Read the model definition and answer for the solid it produces. Units are mm, in the model's axes. Round coordinates to 2 decimals unless told otherwise and drop trailing zeros. Loops run counter-clockwise (first coordinate to the right, second up) from the corner with the lowest first, then second, coordinate; pieces in that order, holes last. Notation, with made-up numbers: M -18.75,54.25 L 32.25,54.25 A11 cw 32.25,69.25 Z; hole C 56,34.25 d9. An arc over 180 degrees is marked long. Answer as CSV lines item,"result".
```python
from build123d import *

# Parameters (mm, degrees)
SKETCH_1_W          = 40
SKETCH_1_H          = 170
SKETCH_1_R          = 1.5
EXTRUDE_1_DEPTH     = 5
FILLET_1_R          = 5
SKETCH_2_R          = 3
CUT_EXTRUDE_1_DEPTH = 3


with BuildPart() as part:
    # 草图1 → 凸台-拉伸1 (new body)
    with BuildSketch(Plane(origin=(0, 0, 0), x_dir=(1, 0, 0), z_dir=(0, 1, 0))):
        Rectangle(SKETCH_1_W, SKETCH_1_H)
        with Locations(Location((-15, 70, 0), (0, 0, 270))):
            Circle(SKETCH_1_R, mode=Mode.SUBTRACT)
        with Locations(Location((15, 70, 0), (0, 0, 270))):
            Circle(SKETCH_1_R, mode=Mode.SUBTRACT)
        with Locations(Location((15, -10, 0), (0, 0, 270))):
            Circle(SKETCH_1_R, mode=Mode.SUBTRACT)
        with Locations(Location((-15, -10, 0), (0, 0, 270))):
            Circle(SKETCH_1_R, mode=Mode.SUBTRACT)
        with Locations(Location((12, -46, 0), (0, 0, 270))):
            Circle(SKETCH_1_R, mode=Mode.SUBTRACT)
        with Locations(Location((-12, -46, 0), (0, 0, 270))):
            Circle(SKETCH_1_R, mode=Mode.SUBTRACT)
        with Locations(Location((-12, -75, 0), (0, 0, 270))):
            Circle(SKETCH_1_R, mode=Mode.SUBTRACT)
        with Locations(Location((12, -75, 0), (0, 0, 270))):
            Circle(SKETCH_1_R, mode=Mode.SUBTRACT)
    extrude(amount=EXTRUDE_1_DEPTH)

    # 圆角1
    fillet_1_edges = [part.edges().sort_by_distance(p)[0] for p in [
        (20, 2.5, 85),
        (-20, 2.5, 85),
        (-20, 2.5, -85),
        (20, 2.5, -85),
    ]]
    fillet(fillet_1_edges, radius=FILLET_1_R)

    # 草图2 → 切除-拉伸1 (cut)
    with BuildSketch(Plane.XZ):
        with Locations(Location((-12, 75, 0), (0, 0, 270))):
            Circle(SKETCH_2_R)
        with Locations(Location((12, 75, 0), (0, 0, 270))):
            Circle(SKETCH_2_R)
        with Locations(Location((12, 46, 0), (0, 0, 270))):
            Circle(SKETCH_2_R)
        with Locations(Location((-12, 46, 0), (0, 0, 270))):
            Circle(SKETCH_2_R)
    extrude(amount=-CUT_EXTRUDE_1_DEPTH, mode=Mode.SUBTRACT)


solid = part.part
```
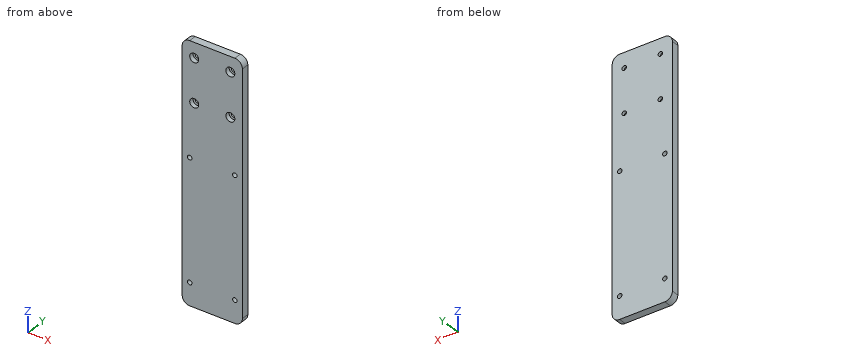
1) This flat-tipped pin is pushed along its axis until it touches: P1, Ø3, axis at x = 12.5, z = 75.5, coming from the -Y side. Where does it stop, or does it pass through?
Evaluation:
P1,"stops at y = 3"
2) Straight lines are drawn through the part: line 1 (Z direction, x = 12, y = 4); line 2 (X direction, y = 2, z = 75); line 3 (Z direction, x = 13, y = 1.85). For each, find the intervals that lie inside material, in ascending order.
Evaluation:
line 1,"z = -85 to 44.5, 47.5 to 73.5, 76.5 to 85"
line 2,"x = -20 to -15, -9 to 9, 15 to 20"
line 3,"z = -85 to 43.17, 48.83 to 72.17, 77.83 to 85"
3) Find section C-C, the plane x = 12. Give the vertices of the cut face in (y, z), then the cut area to 3 significant figures.
Evaluation:
outline,"M 0,-85 L 5,-85 L 5,44.5 L 3,44.5 L 3,43 L 0,43 Z; M 0,49 L 3,49 L 3,47.5 L 5,47.5 L 5,73.5 L 3,73.5 L 3,72 L 0,72 Z; M 0,78 L 3,78 L 3,76.5 L 5,76.5 L 5,85 L 0,85 Z"
area,"802 mm^2"
4) Find section D-D, the plane z = 75. Give the vertices of the cut face in (x, y), then the cut area to 3 significant figures.
Evaluation:
outline,"M -20,0 L -15,0 L -15,3 L -13.5,3 L -13.5,5 L -20,5 Z; M -10.5,3 L -9,3 L -9,0 L 9,0 L 9,3 L 10.5,3 L 10.5,5 L -10.5,5 Z; M 13.5,3 L 15,3 L 15,0 L 20,0 L 20,5 L 13.5,5 Z"
area,"152 mm^2"
5) Find section B-B, the plane y = 1.25. Count the separate pieces of the cut face and the enclosed holes in it, then the cut area to 3 significant figures.
Evaluation:
separate pieces,"1"
enclosed holes,"8"
area,"6,640 mm^2"
6) Find section A-A, the plane z = 10. Give the vertices of the cut face in (x, y).
Evaluation:
outline,"M -20,0 L -16.5,0 L -16.5,5 L -20,5 Z; M -13.5,0 L 13.5,0 L 13.5,5 L -13.5,5 Z; M 16.5,0 L 20,0 L 20,5 L 16.5,5 Z"
